Verification items for this drawing (mm, ordinates from the low corner). A direction names the side the tool comes from. Give positions to 0.01 mm unless a question says otherwise; leave off trailing zeros. Write each loop counter-clockwise with the first axis right and the second up, starting at its lowest first coordinate (ties: lowest second). Pieces come first, ordered by that corner, then holes. Notation, with made-up numbers: M 77,6 L 113,6 A29 ccw 113,33 Z; hole C 30.25,61 d10. An arc over 180 degrees is marked long. Write each question's results on one line, items separated by ' | '.
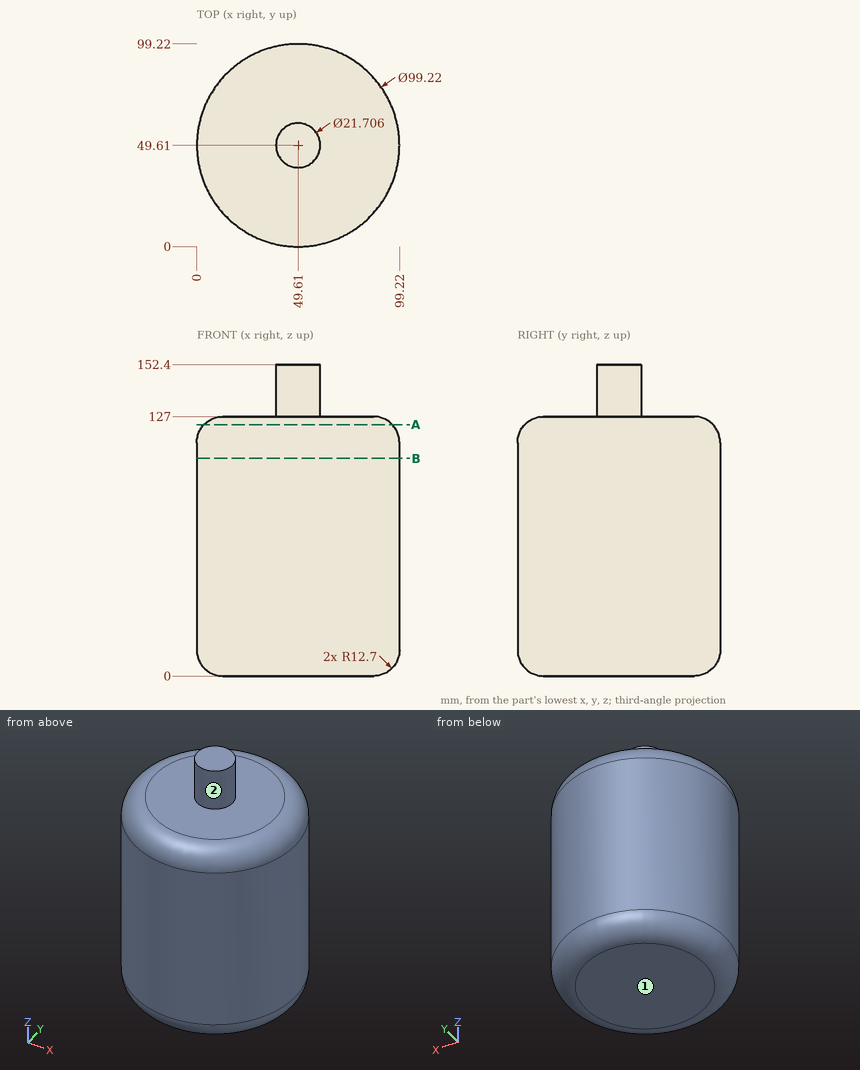
Q1. Section check B-B (z = 106.5). Enter the section's corners in (x, y), then the cut area to 3 significant figures.
Answer key:
outline: C 49.61,49.61 d99.22 | area: 7,730 mm2
Q2. Material ranges on probe 1 along Z at (x, y) = (79, 55); probe 2 along Z at (x, y) = (4.5, 46.5) (1 decimal); probe 3 along Y at (x, z) = (9, 27) (1 decimal), recorded low to high. Write a range as [from, to].
Answer key:
probe 1: z = [0, 127] | probe 2: z = [3.1, 123.9] | probe 3: y = [21.1, 78.1]
Q3. Access from +Z, -Z, +X, -X, +Y, -Y to the whole of each face (thin tool, end or side, straight path). Record for the marked faces 1 and 2.
Answer key:
face 1: -Z, +X, -X, +Y, -Y | face 2: +Z
Q4. Depth check by flat-ended pin: P1, Ø5, axis at y = 67, z = 32.5, coming from the +X side; P2, Ø1, axis at x = 72, z = 60, coming from the -Y side; P3, Ø8, axis at x = 84.5, z = 78.5, coming from the -Y side. Enter the tip coordinate at first touch or a pass-through.
Answer key:
P1: stops at x = 96.93 | P2: stops at y = 5.09 | P3: stops at y = 10.79
Q5. Section check A-A (z = 123). Enter the section's corners in (x, y), then the cut area to 3 significant figures.
Answer key:
outline: C 49.61,49.61 d92.32 | area: 6,690 mm2
